```python
from build123d import *

# Parameters (mm, degrees)
SKETCH1_R           = 37
SKETCH1_R_2         = 35
BOSS_EXTRUDE1_DEPTH = 98.5
CUT_EXTRUDE2_REACH  = 76
CUT_EXTRUDE3_DEPTH  = 5
BOSS_EXTRUDE2_DEPTH = 42
CIRPATTERN1_COUNT   = 6


with BuildPart() as part:
    # Sketch1 → Boss-Extrude1 (new body)
    with BuildSketch(Plane(origin=(0, 0, 0), x_dir=(1, 0, 0), z_dir=(0, 1, 0))):
        Circle(SKETCH1_R)
        Circle(SKETCH1_R_2, mode=Mode.SUBTRACT)
    extrude(amount=BOSS_EXTRUDE1_DEPTH)

    # Sketch2 → Cut-Extrude2 (cut, up to next)
    with BuildSketch(Plane.XY.offset(37), mode=Mode.PRIVATE) as cut_extrude2_sk1:
        with BuildLine():
            Line((-8.45, 0), (-4.916814722, 17))
            ThreePointArc((-4.916814722, 17), (0, 21), (4.916814722, 17))
            Line((4.916814722, 17), (8.45, 0))
            Line((8.45, 0), (-8.45, 0))
        make_face()
    cut_extrude2_tool1 = extrude(cut_extrude2_sk1.sketch, amount=-CUT_EXTRUDE2_REACH, mode=Mode.PRIVATE) & part.part
    add(cut_extrude2_tool1.solids().sort_by_distance((0, 9.002939, 37))[0], mode=Mode.SUBTRACT)

    # Sketch4 → Cut-Extrude3 (cut)
    with BuildSketch(Plane(origin=(0, 98.5, 0), x_dir=(1, 0, 0), z_dir=(0, 1, 0))):
        with BuildLine():
            Line((20.172972973, -28.601593687), (21.325714286, -30.235970469))
            ThreePointArc((21.325714286, -30.235970469), (9.649317719, -35.719611806), (-3.2, -36.861361885))
            Line((-3.2, -36.861361885), (-3.027027027, -34.868855837))
            ThreePointArc((-3.027027027, -34.868855837), (9.127732978, -33.788821978), (20.172972973, -28.601593687))
        make_face()
    extrude(amount=-CUT_EXTRUDE3_DEPTH, mode=Mode.SUBTRACT)

    # Sketch5 → Boss-Extrude2 (add)
    with BuildSketch(Plane(origin=(0, 33, 0), x_dir=(1, 0, 0), z_dir=(0, 1, 0))):
        with BuildLine():
            Line((-12.5, -32.691742077), (-10, -26.153393661))
            ThreePointArc((-10, -26.153393661), (0, -28), (10, -26.153393661))
            Line((10, -26.153393661), (12.5, -32.691742077))
            ThreePointArc((12.5, -32.691742077), (0, -35), (-12.5, -32.691742077))
        make_face()
    boss_extrude2 = extrude(amount=BOSS_EXTRUDE2_DEPTH)

    # CirPattern1: Boss-Extrude2 ×6 about axis
    cirpattern1_axis = Axis((0, 0, 0), (0, 1, 0))
    for i in range(1, CIRPATTERN1_COUNT):
        add(boss_extrude2.rotate(cirpattern1_axis, i * 360 / CIRPATTERN1_COUNT))


solid = part.part
```
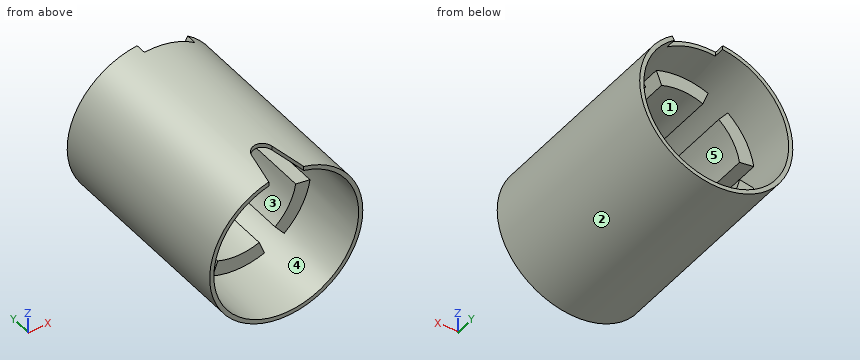
Verification items for the finished model (mm, model axes). Face numbers are marked on the shaded views. A direction names the side the tool comes from. Round coordinates to 2 decimals unless told otherwise and drop trailing zeros. Loops run counter-clockwise (first coordinate to the right, second up) from the corner with the lowest first, then second, coordinate; pieces in that order, holes last. Notation, with made-up numbers: (14, 29) -> (67, 29) arc R31 ccw to (67, 59) -> close; hole circle Ø1 at (69, 10). An arc over 180 degrees is marked (long way). Answer as a JSON object with one key per item and string values.
Q1. Go/stop test with flat-tipped pins: P1, Ø8.5, axis at x = -25, z = -15.5, coming from the +Y side; P2, Ø1.5, axis at x = 27.5, y = 86, coming from the +Z side; P3, Ø3, axis at y = 40, z = -16, coming from the +X side. Record where each tip stops, or that it passes through.
Data:
{"P1": "stops at y = 75", "P2": "stops at z = 25.56", "P3": "stops at x = 34.04"}
Q2. Draft check along Z on the marked faces 1, 2 and 3. Enter one of: pulls with the +Z half, pulls with the -Z half, needs draft (parallel to the pull), parting line crosses it, or undercut.
Data:
{"face 1": "undercut", "face 2": "parting line crosses it", "face 3": "undercut"}
Q3. Section check B-B (z = 0). Record the boundary of the cut face in (x, y).
Data:
{"outline": "(-37, 0) -> (-35, 0) -> (-35, 98.5) -> (-37, 98.5) -> close; (35, 0) -> (37, 0) -> (37, 98.5) -> (35, 98.5) -> close"}
Q4. Section check C-C (y = 55). Record the boundary of the cut face in (x, z), then the cut area to 3 significant figures.
Data:
{"outline": "circle Ø74 at (0, 0); hole (-34.56, -5.52) -> (-27.65, -4.42) arc R28 ccw to (-17.65, -21.74) -> (-22.06, -27.17) arc R35 ccw to (-12.5, -32.69) -> (-10, -26.15) arc R28 ccw to (10, -26.15) -> (12.5, -32.69) arc R35 ccw to (22.06, -27.17) -> (17.65, -21.74) arc R28 ccw to (27.65, -4.42) -> (34.56, -5.52) arc R35 ccw to (34.56, 5.52) -> (27.65, 4.42) arc R28 ccw to (17.65, 21.74) -> (22.06, 27.17) arc R35 ccw to (12.5, 32.69) -> (10, 26.15) arc R28 ccw to (-10, 26.15) -> (-12.5, 32.69) arc R35 ccw to (-22.06, 27.17) -> (-17.65, 21.74) arc R28 ccw to (-27.65, 4.42) -> (-34.56, 5.52) arc R35 ccw to start", "area": "1,420 mm2"}
Q5. Section check D-D (x = -20). Record the boundary of the cut face in (y, z), then the cut area to 3 significant figures.
Data:
{"outline": "(0, -31.13) -> (98.5, -31.13) -> (98.5, -28.72) -> (0, -28.72) -> close; (0, 28.72) -> (98.5, 28.72) -> (98.5, 31.13) -> (0, 31.13) -> close; (33, -24.63) -> (75, -24.63) -> (75, -19.6) -> (33, -19.6) -> close; (33, 19.6) -> (75, 19.6) -> (75, 24.63) -> (33, 24.63) -> close", "area": "897 mm2"}
Q6. Access from +Z, -Z, +X, -X, +Y, -Y to the whole of each face (thin tool, end or side, straight path). Record for the marked faces 4 and 5.
Data:
{"face 4": "none", "face 5": "+Y, -Y"}
Q7. Scan lines: line 1 (X direction, y = 63.5, z = 0); line 2 (Z direction, x = 0, y = 49). Record each from-to range of solid material in increasing order. Write a range as from..to.
Data:
{"line 1": "x = -37..-35, 35..37", "line 2": "z = -37..-28, 28..37"}
Q8. Section check A-A (x = 0). Record the boundary of the cut face in (y, z).
Data:
{"outline": "(0, -37) -> (98.5, -37) -> (98.5, -35) -> (75, -35) -> (75, -28) -> (33, -28) -> (33, -35) -> (0, -35) -> close; (21, 35) -> (33, 35) -> (33, 28) -> (75, 28) -> (75, 35) -> (93.5, 35) -> (93.5, 37) -> (21, 37) -> close"}
